Here's the drawing with two shaded views (mm, measured from the low corner). I have some questions. A direction names the side the tool comes from. Give positions to 0.01 mm unless a question says otherwise; leave off trailing zeros. Write each loop counter-clockwise with the first axis right and the second up, starting at its lowest first coordinate (ties: lowest second). Pieces come first, ordered by that corner, then holes. Notation, with made-up numbers: M 54,54.25 L 82,54.25 A21 cw 82,62.25 Z; hole C -33,32.25 d4. An arc over 180 degrees is marked long. Use one line per item in the form item = value. Start each with the question number.
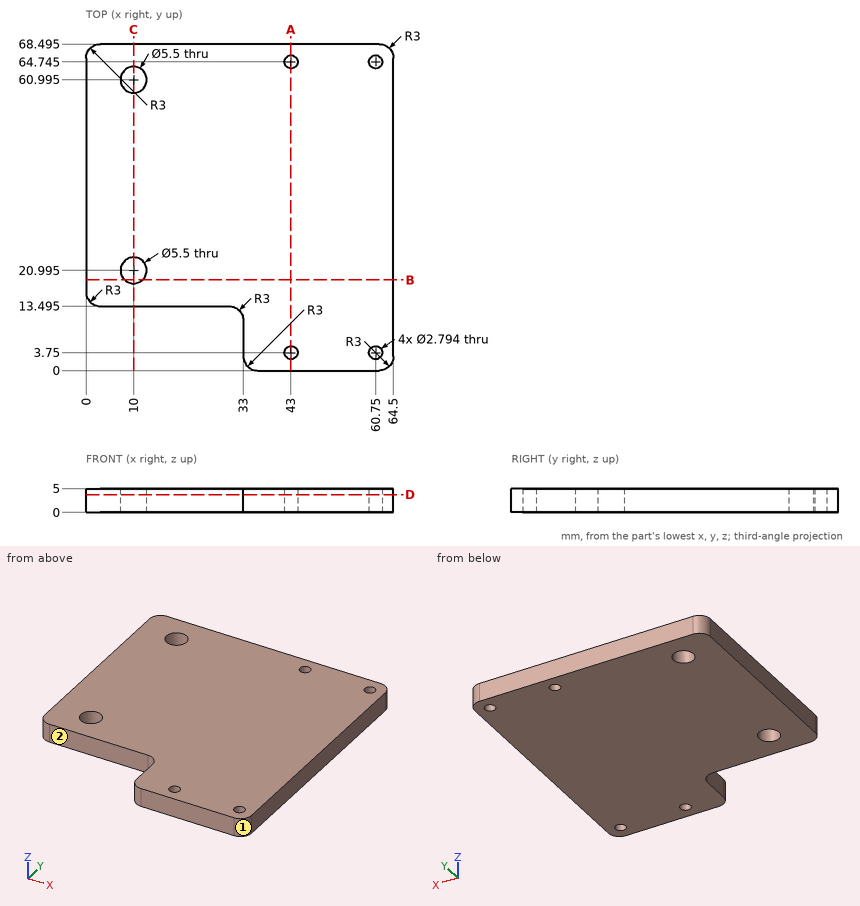
1) Suppose I cut it at A-A, the plane x = 43. List the corners of the cut face in (y, z) for me (3 decimals).
2) Please list where these lines run through material, in increasing order: line 1 (Y direction, x = 43, z = 2.7) (3 decimals); line 2 (Y direction, x = 10.5, z = 2.4) (3 decimals); line 3 (Y direction, x = 13, z = 2.45) (3 decimals).
3) Suppose I cut it at D-D, the plane z = 3.7. List the corners of the cut face in (x, y) for me (3 decimals).
4) On a 3-axis mill with a long thin cutter (end or side, diameter ignored), from which of +Z, -Z, +X, -X, +Y, -Y can I reach the whole of each face in a straight line? I mean the marked faces 1 and 2. Say none if no direction works.
5) Suppose I cut it at C-C, the plane x = 10. List the corners of the cut face in (y, z) for me (3 decimals).
6) Suppose I cut it at B-B, the plane y = 19. List the corners of the cut face in (x, z) for me.
7) Will this pin go through, and if not, where does the flat tip stop? P1, Ø1.7, axis at x = 60.75, y = 3.75, coming from the -Z side.
Checks:
q1.outline = M 0,0 L 2.353,0 L 2.353,5 L 0,5 Z; M 5.147,0 L 63.348,0 L 63.348,5 L 5.147,5 Z; M 66.142,0 L 68.495,0 L 68.495,5 L 66.142,5 Z
q2.line_1 = 0 to 2.353, 5.147 to 63.348, 66.142 to 68.495
q2.line_2 = 13.495 to 18.291, 23.699 to 58.291, 63.699 to 68.495
q2.line_3 = 13.495 to 68.495
q3.outline = M 0,16.495 A3 ccw 3,13.495 L 30,13.495 A3 cw 33,10.495 L 33,3 A3 ccw 36,0 L 61.5,0 A3 ccw 64.5,3 L 64.5,65.495 A3 ccw 61.5,68.495 L 3,68.495 A3 ccw 0,65.495 Z; hole C 10,20.995 d5.5; hole C 10,60.995 d5.5; hole C 43,3.75 d2.794; hole C 43,64.745 d2.794; hole C 60.75,3.75 d2.794; hole C 60.75,64.745 d2.794
q4.face_1 = +Z, -Z, +X, -Y
q4.face_2 = +Z, -Z, -X, -Y
q5.outline = M 13.495,0 L 18.245,0 L 18.245,5 L 13.495,5 Z; M 23.745,0 L 58.245,0 L 58.245,5 L 23.745,5 Z; M 63.745,0 L 68.495,0 L 68.495,5 L 63.745,5 Z
q6.outline = M 0,0 L 8.11,0 L 8.11,5 L 0,5 Z; M 11.89,0 L 64.5,0 L 64.5,5 L 11.89,5 Z
q7.P1 = through
